Geometry: final body of the model. Coordinates: model frame, mm. A direction names the side the tool comes from. Give positions to 0.01 mm unless a question says otherwise; leave off trailing zeros. Write each loop counter-clockwise with the first axis right and the second up, starting at its lowest first coordinate (ties: lowest second). Pieces come first, ordered by that corner, then holes.
Q1. Draft query along X for faces 6 (the face through (1.57, 33.32, 1.57)), 7 (the face through (46, 53.975, -80)), 8 (the face through (83.74, 15.01, -79.8)). Return one class per face: pulls with the +X half, pulls with the -X half, needs draft (parallel to the pull), parting line crosses it, or undercut.
Q2. Cut plane B-B on x = 77. Return the cut outline in (y, z) (3 decimals).
Q3. Reachability of faces 1 (the face through (90.637, 33.315, 1.565)), 2 (the face through (45, 29, -81.407)), 3 (the face through (45, 19, 0)), 4 (the face through (46, 34.925, 2)), 5 (the face through (92.202, 3, -42)) from +Z, -Z, +X, -X, +Y, -Y: full face, straight path, thin tool, end or side. Return the list, or none.
Q4. Cut plane D-D on z = -38. Return the cut outline in (x, y) (3 decimals).
Q5. Cut plane C-C on y = 48. Return the cut outline in (x, z), plus the area to 3 significant figures.
Q6. Line query: L1, parallel to Z at x = 58, y = 23.5 (3 decimals); L2, parallel to Y at x = 65.5, z = -8.5 (3 decimals); L3, parallel to Z at x = 5.5, y = 35. Output: solid intervals per line, ascending.
Q7. Cut plane A-A on y = 21. Return the cut outline in (x, z) (3 decimals).
Q8. Pin query (flat end, axial travel): pin 1 (8.5 mm diameter, centred on x = 85.852, y = 16.637, fed in from -Z); pin 2 (10 mm diameter, centred on y = 8.5, z = -31, fed in from +X); pin 3 (1.6 mm diameter, centred on x = 47.5, z = 2, fed in from +Y) (3 decimals); pin 4 (1 mm diameter, centred on x = 42.5, z = -31, fed in from +Y) (3 decimals). Return the tip coordinate at first contact, or that it passes through.
```python
from build123d import *

# Parameters (mm, degrees)
SKETCH1_W            = 92.202
SKETCH1_H            = 78.232
BOSS_EXTRUDE1_DEPTH  = 3.175
EDGE_FLANGE1_DEPTH   = 92.202
EDGE_FLANGE1_2_DEPTH = 92.202
EDGE_FLANGE2_DEPTH   = 92.202
EDGE_FLANGE2_2_DEPTH = 92.202
SKETCH9_R            = 2.667
CUT_EXTRUDE1_DEPTH   = 137.266738983
CHAMFER1_SIZE        = 3.175


# Read off the part's stored shape, not the designer's step: Edge-Flange1, Edge-Flange2
with BuildPart() as part:
    # Sketch1 → Boss-Extrude1 (new body)
    with BuildSketch(Plane(origin=(0, 0, 0), x_dir=(1, 0, 0), z_dir=(0, 1, 0))):
        with Locations((46.101, 39.116)):
            Rectangle(SKETCH1_W, SKETCH1_H)
    extrude(amount=BOSS_EXTRUDE1_DEPTH)

    # Edge-Flange1 outline → Edge-Flange1 (cut)
    with BuildSketch(Plane.YZ):
        with BuildLine():
            Line((0, -78.232), (0.074445793, -78.232))
            ThreePointArc((0.074445793, -78.232), (0.018655648, -77.852813981), (0, -77.47))
            Line((0, -77.47), (0, -78.232))
        make_face()
    extrude(amount=EDGE_FLANGE1_DEPTH, mode=Mode.SUBTRACT)

    # Edge-Flange1 2 outline → Edge-Flange1 2 (add)
    with BuildSketch(Plane.YZ):
        with BuildLine():
            ThreePointArc((0.074445793, -78.232), (1.4370025, -80.511378224), (3.937, -81.407))
            Line((3.937, -81.407), (53.975, -81.407))
            Line((53.975, -81.407), (53.975, -78.232))
            Line((53.975, -78.232), (3.937, -78.232))
            ThreePointArc((3.937, -78.232), (3.398184633, -78.008815367), (3.175, -77.47))
            Line((3.175, -77.47), (3.175, -78.232))
            Line((3.175, -78.232), (0.074445793, -78.232))
        make_face()
    extrude(amount=EDGE_FLANGE1_2_DEPTH)

    # Edge-Flange2 outline → Edge-Flange2 (cut)
    with BuildSketch(Plane.YZ):
        with BuildLine():
            ThreePointArc((0, -0.762), (0.018655648, -0.379186019), (0.074445793, 0))
            Line((0.074445793, 0), (0, 0))
            Line((0, 0), (0, -0.762))
        make_face()
    extrude(amount=EDGE_FLANGE2_DEPTH, mode=Mode.SUBTRACT)

    # Edge-Flange2 2 outline → Edge-Flange2 2 (add)
    with BuildSketch(Plane.YZ):
        with BuildLine():
            Line((34.925, 3.175), (3.937, 3.175))
            ThreePointArc((3.937, 3.175), (1.4370025, 2.279378224), (0.074445793, 0))
            Line((0.074445793, 0), (3.175, 0))
            Line((3.175, 0), (3.175, -0.762))
            ThreePointArc((3.175, -0.762), (3.398184633, -0.223184633), (3.937, 0))
            Line((3.937, 0), (34.925, 0))
            Line((34.925, 0), (34.925, 3.175))
        make_face()
    extrude(amount=EDGE_FLANGE2_2_DEPTH)

    # Sketch9 → Cut-Extrude1 (cut, through all)
    with BuildSketch(Plane.XY.offset(3.175)):
        with Locations((85.852, 16.637)):
            Circle(SKETCH9_R)
    extrude(amount=-CUT_EXTRUDE1_DEPTH, mode=Mode.SUBTRACT)

    # Chamfer1
    chamfer1_edges = [part.edges().sort_by_distance(p)[0] for p in [
        (92.202, 53.975, -79.8195),
        (0, 53.975, -79.8195),
        (0, 34.925, 1.5875),
        (92.202, 34.925, 1.5875),
    ]]
    chamfer(chamfer1_edges, length=CHAMFER1_SIZE)


solid = part.part
```
Data:
1. face 6: pulls with the -X half
1. face 7: needs draft
1. face 8: undercut
2. outline: (0, -77.47) arc R3.937 ccw to (3.937, -81.407) - (53.975, -81.407) - (53.975, -78.232) - (3.937, -78.232) arc R0.762 cw to (3.175, -77.47) - (3.175, -0.762) arc R0.762 cw to (3.937, 0) - (34.925, 0) - (34.925, 3.175) - (3.937, 3.175) arc R3.937 ccw to (0, -0.762) - close
3. face 1: +Z, +X, +Y
3. face 2: -Z, +X, -X, +Y, -Y
3. face 3: +X, -X, +Y
3. face 4: +Z, +X, -X, +Y
3. face 5: +Z, -Z, +X, +Y, -Y
4. outline: (0, 0) - (92.202, 0) - (92.202, 3.175) - (0, 3.175) - close
5. outline: (0, -81.41) - (92.2, -81.41) - (92.2, -78.23) - (0, -78.23) - close
5. area: 293 mm2
6. L1: z = -81.407 to -78.232, 0 to 3.175
6. L2: y = 0 to 3.175
6. L3: z = -81.41 to -78.23
7. outline: (0, -81.407) - (92.202, -81.407) - (92.202, -78.232) - (0, -78.232) - close; (0, 0) - (92.202, 0) - (92.202, 3.175) - (0, 3.175) - close
8. pin 1: stops at z = -81.41
8. pin 2: passes through
8. pin 3: stops at y = 34.925
8. pin 4: stops at y = 3.175
